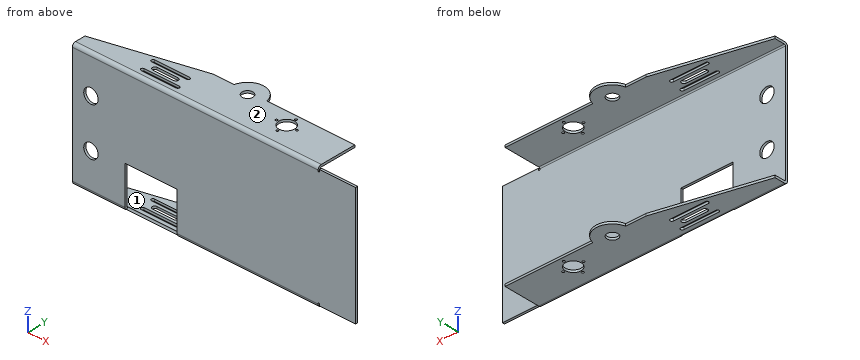
from build123d import *

# Parameters (mm, degrees)
SKETCH3_W                       = 250
SKETCH3_H                       = 105
SKETCH3_R                       = 6.35
BASE_FLANGE1_DEPTH              = 2
EDGE_FLANGE1_STRIP_W            = 10
EDGE_FLANGE1_STRIP_H            = 2
EDGE_FLANGE1_STRIP_CUT_DEPTH    = 217
EDGE_FLANGE1_RELIEF_W           = 11
EDGE_FLANGE1_RELIEF_H           = 1
EDGE_FLANGE1_RELIEF_CUT_DEPTH   = 2
EDGE_FLANGE1_STRIP_2_W          = 10
EDGE_FLANGE1_STRIP_2_H          = 2
EDGE_FLANGE1_STRIP_CUT_2_DEPTH  = 217
EDGE_FLANGE1_RELIEF_2_W         = 11
EDGE_FLANGE1_RELIEF_2_H         = 1
EDGE_FLANGE1_RELIEF_CUT_2_DEPTH = 2
EDGE_FLANGE1_DEPTH              = 217
EDGE_FLANGE1_START              = 2
EDGE_FLANGE1_PROFILE_R          = 4.7625
EDGE_FLANGE1_FLAT_DEPTH         = 2
EDGE_FLANGE1_BEND_DEPTH         = 217
EDGE_FLANGE1_PROFILE_2_R        = 4.7625
EDGE_FLANGE1_FLAT_2_DEPTH       = 2
CUT_EXTRUDE2_START              = -78.75
CUT_EXTRUDE2_DEPTH              = 46.25
CUT_EXTRUDE1_DEPTH              = 144.523278273
CUT_EXTRUDE1_DEPTH_BACK         = 144.523278273
SKETCH14_R                      = 1
SKETCH14_R_2                    = 7


# Read off the part's stored shape, not the designer's step: Cut-Extrude2
# Sheet-metal steps are written as plain solids
with BuildPart() as part:
    # Sketch3 → Base-Flange1 (new body)
    with BuildSketch(Plane(origin=(0, 0, 0), x_dir=(1, 0, 0), z_dir=(0, 1, 0))):
        Rectangle(SKETCH3_W, SKETCH3_H)
        with Locations(Location((-108.65, 21.15, 0), (0, 0, 270))):
            Circle(SKETCH3_R, mode=Mode.SUBTRACT)
        with Locations(Location((-108.65, -21.15, 0), (0, 0, 90))):
            Circle(SKETCH3_R, mode=Mode.SUBTRACT)
    extrude(amount=-BASE_FLANGE1_DEPTH)

    # Edge-Flange1 strip (across the edge) → Edge-Flange1 strip cut (cut)
    with BuildSketch(Plane(origin=(-125, 0, 52.5), x_dir=(0, 0, -1), z_dir=(1, 0, 0))):
        with Locations((-4, -1)):
            Rectangle(EDGE_FLANGE1_STRIP_W, EDGE_FLANGE1_STRIP_H)
    extrude(amount=EDGE_FLANGE1_STRIP_CUT_DEPTH, mode=Mode.SUBTRACT)

    # Edge-Flange1 relief (on the sheet) → Edge-Flange1 relief cut (cut)
    with BuildSketch(Plane(origin=(-125, 0, 51.5), x_dir=(0, 0, -1), z_dir=(0, 1, 0))):
        with Locations((-4.5, -217.5)):
            Rectangle(EDGE_FLANGE1_RELIEF_W, EDGE_FLANGE1_RELIEF_H)
    extrude(amount=-EDGE_FLANGE1_RELIEF_CUT_DEPTH, mode=Mode.SUBTRACT)

    # Edge-Flange1 strip 2 (across the edge) → Edge-Flange1 strip cut 2 (cut)
    with BuildSketch(Plane(origin=(92, 0, -52.5), x_dir=(0, 0, 1), z_dir=(-1, 0, 0))):
        with Locations((-4, -1)):
            Rectangle(EDGE_FLANGE1_STRIP_2_W, EDGE_FLANGE1_STRIP_2_H)
    extrude(amount=EDGE_FLANGE1_STRIP_CUT_2_DEPTH, mode=Mode.SUBTRACT)

    # Edge-Flange1 relief 2 (on the sheet) → Edge-Flange1 relief cut 2 (cut)
    with BuildSketch(Plane(origin=(92, 0, -51.5), x_dir=(0, 0, 1), z_dir=(0, 1, 0))):
        with Locations((-4.5, 0.5)):
            Rectangle(EDGE_FLANGE1_RELIEF_2_W, EDGE_FLANGE1_RELIEF_2_H)
    extrude(amount=-EDGE_FLANGE1_RELIEF_CUT_2_DEPTH, mode=Mode.SUBTRACT)

    # Edge-Flange1 bend section (across the edge) → Edge-Flange1 (add)
    with BuildSketch(Plane(origin=(-125, 0, 52.5), x_dir=(0, 0, -1), z_dir=(1, 0, 0))):
        with BuildLine():
            Line((-2, 1), (0, 1))
            ThreePointArc((0, 1), (0.292893219, 0.292893219), (1, 0))
            Line((1, 0), (1, -2))
            ThreePointArc((1, -2), (-1.121320344, -1.121320344), (-2, 1))
        make_face()
    extrude(amount=EDGE_FLANGE1_DEPTH)

    # Edge-Flange1 profile (on flange) → Edge-Flange1 flat (add)
    with BuildSketch(Plane.XY.offset(52.5).offset(EDGE_FLANGE1_START)):
        with BuildLine():
            Line((-125, 9.993471807), (-125, 1))
            Line((-125, 1), (92, 1))
            Line((92, 1), (92, 33))
            Line((92, 33), (14.454459736, 33))
            ThreePointArc((14.454459736, 33), (0, 44.7625), (-14.454459736, 33))
            Line((-14.454459736, 33), (-32.5, 33))
            Line((-32.5, 33), (-125, 9.993471807))
        make_face()
        with Locations((0, 30)):
            Circle(EDGE_FLANGE1_PROFILE_R, mode=Mode.SUBTRACT)
    extrude(amount=-EDGE_FLANGE1_FLAT_DEPTH)

    # Edge-Flange1 bend section 2 (across the edge) → Edge-Flange1 bend (add)
    with BuildSketch(Plane(origin=(92, 0, -52.5), x_dir=(0, 0, 1), z_dir=(-1, 0, 0))):
        with BuildLine():
            Line((-2, 1), (0, 1))
            ThreePointArc((0, 1), (0.292893219, 0.292893219), (1, 0))
            Line((1, 0), (1, -2))
            ThreePointArc((1, -2), (-1.121320344, -1.121320344), (-2, 1))
        make_face()
    extrude(amount=EDGE_FLANGE1_BEND_DEPTH)

    # Edge-Flange1 profile 2 (on flange) → Edge-Flange1 flat 2 (add)
    with BuildSketch(Plane(origin=(0, 0, -52.5), x_dir=(-1, 0, 0), z_dir=(0, 0, -1)).offset(EDGE_FLANGE1_START)):
        with BuildLine():
            ThreePointArc((14.454459736, 33), (0, 44.7625), (-14.454459736, 33))
            Line((-14.454459736, 33), (-92, 33))
            Line((-92, 33), (-92, 1))
            Line((-92, 1), (125, 1))
            Line((125, 1), (125, 9.993471807))
            Line((125, 9.993471807), (32.5, 33))
            Line((32.5, 33), (14.454459736, 33))
        make_face()
        with Locations((0, 30)):
            Circle(EDGE_FLANGE1_PROFILE_2_R, mode=Mode.SUBTRACT)
    extrude(amount=-EDGE_FLANGE1_FLAT_2_DEPTH)

    # Cut-Extrude2 outline → Cut-Extrude2 (cut)
    with BuildSketch(Plane.YZ.offset(CUT_EXTRUDE2_START)):
        with BuildLine():
            Line((0, -54.328427125), (0.666666667, -52.442809042))
            ThreePointArc((0.666666667, -52.442809042), (0.183503419, -52.077350269), (0, -51.5))
            Line((0, -51.5), (0, -17.5))
            Line((0, -17.5), (-2, -17.5))
            Line((-2, -17.5), (-2, -51.5))
            ThreePointArc((-2, -51.5), (-1.449489743, -53.232050808), (0, -54.328427125))
        make_face()
    extrude(amount=CUT_EXTRUDE2_DEPTH, mode=Mode.SUBTRACT)

    # Sketch14 → Cut-Extrude1 (cut, two sides: drawn at the far end of the back side and taken through both)
    with BuildSketch(Plane.XY.offset(-CUT_EXTRUDE1_DEPTH_BACK)):
        with BuildLine():
            Line((-46.5, 14.125), (-65.166666667, 14.125))
            ThreePointArc((-65.166666667, 14.125), (-67.291666667, 12), (-65.166666667, 9.875))
            Line((-65.166666667, 9.875), (-46.5, 9.875))
            ThreePointArc((-46.5, 9.875), (-44.375, 12), (-46.5, 14.125))
        make_face()
        with BuildLine():
            Line((-57.900010285, 4.380710415), (-51.653085966, 4.380710415))
            ThreePointArc((-51.653085966, 4.380710415), (-50.153085966, 5.880710415), (-51.653085966, 7.380710415))
            Line((-51.653085966, 7.380710415), (-57.900010285, 7.380710415))
            ThreePointArc((-57.900010285, 7.380710415), (-59.400010285, 5.880710415), (-57.900010285, 4.380710415))
        make_face()
        with BuildLine():
            Line((-51.653085966, 4.380710415), (-39.233343618, 4.380710415))
            ThreePointArc((-39.233343618, 4.380710415), (-37.733343618, 5.880710415), (-39.233343618, 7.380710415))
            Line((-39.233343618, 7.380710415), (-51.653085966, 7.380710415))
            ThreePointArc((-51.653085966, 7.380710415), (-50.153085966, 5.880710415), (-51.653085966, 4.380710415))
        make_face()
        with BuildLine():
            Line((-70.319752633, 4.380710415), (-57.900010285, 4.380710415))
            ThreePointArc((-57.900010285, 4.380710415), (-59.400010285, 5.880710415), (-57.900010285, 7.380710415))
            Line((-57.900010285, 7.380710415), (-70.319752633, 7.380710415))
            ThreePointArc((-70.319752633, 7.380710415), (-71.819752633, 5.880710415), (-70.319752633, 4.380710415))
        make_face()
        with BuildLine():
            Line((-72.433323049, 16.619289585), (-60.0135807, 16.619289585))
            ThreePointArc((-60.0135807, 16.619289585), (-61.5135807, 18.119289585), (-60.0135807, 19.619289585))
            Line((-60.0135807, 19.619289585), (-72.433323049, 19.619289585))
            ThreePointArc((-72.433323049, 19.619289585), (-73.933323049, 18.119289585), (-72.433323049, 16.619289585))
        make_face()
        with BuildLine():
            Line((-60.0135807, 16.619289585), (-53.766656382, 16.619289585))
            ThreePointArc((-53.766656382, 16.619289585), (-52.266656382, 18.119289585), (-53.766656382, 19.619289585))
            Line((-53.766656382, 19.619289585), (-60.0135807, 19.619289585))
            ThreePointArc((-60.0135807, 19.619289585), (-61.5135807, 18.119289585), (-60.0135807, 16.619289585))
        make_face()
        with BuildLine():
            ThreePointArc((-53.766656382, 19.619289585), (-52.266656382, 18.119289585), (-53.766656382, 16.619289585))
            Line((-53.766656382, 16.619289585), (-41.346914034, 16.619289585))
            ThreePointArc((-41.346914034, 16.619289585), (-39.846914034, 18.119289585), (-41.346914034, 19.619289585))
            Line((-41.346914034, 19.619289585), (-53.766656382, 19.619289585))
        make_face()
        with Locations((43.5, 11.4)):
            Circle(SKETCH14_R)
        with Locations((52.5, 20.4)):
            Circle(SKETCH14_R)
        with Locations((43.5, 20.4)):
            Circle(SKETCH14_R_2)
        with Locations((34.5, 20.4)):
            Circle(SKETCH14_R)
        with Locations((43.5, 29.4)):
            Circle(SKETCH14_R)
    extrude(amount=CUT_EXTRUDE1_DEPTH + CUT_EXTRUDE1_DEPTH_BACK, mode=Mode.SUBTRACT)


solid = part.part
The listing builds one solid part. Answer for the finished solid, in the listing's coordinates (mm). Face numbers are marked on the shaded views. A direction names the side the tool comes from. Give positions to 0.01 mm unless a question says otherwise; leave off trailing zeros. Write each loop counter-clockwise with the first axis right and the second up, starting at its lowest first coordinate (ties: lowest second). Pieces come first, ordered by that corner, then holes.
1) Section A-A (z = -21.15) is taken. Write down the section's boundary in (x, y), and give its area (3 significant figures).
2) Section C-C (x = 0) is taken. Write down the section's boundary in (y, z).
3) Section D-D (z = -38.5) is taken. Write down the section's boundary in (x, y).
4) Find the intervals of material crossed by L1, parallel to X at y = -0.5, z = 21.15; L2, parallel to Z at x = -2.5, y = 36.5; L3, parallel to Y at x = -15.5, z = 11.5, in increasing order.
5) A tool of negligible diameter and unlimited length cuts with its end or side. For the marked faces 1 and 2, from which of +Z, -Z, +X, -X, +Y, -Y can it reach the whole face along a straight path? Write none if from no direction.
6) Given P1, Ø4.5, axis at y = 22.5, z = -52.5, coming from the +X side; P2, Ø1.6, axis at x = -58, z = -54, coming from the +Y side; P3, Ø1, axis at x = -53.5, z = -53, coming from the -Y side, each flat-ended and moving along its own axis, determine where each tip first touches the part or whether it passes through.
7) Section B-B (z = 21.15) is taken. Write down the section's boundary in (x, y), and give its area (3 significant figures).
Response:
1. outline: (-125, -2) - (-115, -2) - (-115, 0) - (-125, 0) - close; (-102.3, -2) - (-78.75, -2) - (-78.75, 0) - (-102.3, 0) - close; (-32.5, -2) - (125, -2) - (125, 0) - (-32.5, 0) - close
1. area: 382 mm2
2. outline: (-2, -51.5) arc R3 ccw to (1, -54.5) - (25.24, -54.5) - (25.24, -52.5) - (1, -52.5) arc R1 cw to (0, -51.5) - (0, 51.5) arc R1 cw to (1, 52.5) - (25.24, 52.5) - (25.24, 54.5) - (1, 54.5) arc R3 ccw to (-2, 51.5) - close; (34.76, -54.5) - (44.76, -54.5) - (44.76, -52.5) - (34.76, -52.5) - close; (34.76, 52.5) - (44.76, 52.5) - (44.76, 54.5) - (34.76, 54.5) - close
3. outline: (-125, -2) - (-78.75, -2) - (-78.75, 0) - (-125, 0) - close; (-32.5, -2) - (125, -2) - (125, 0) - (-32.5, 0) - close
4. L1: x = -125 to -115, -102.3 to 125
4. L2: z = -54.5 to -52.5, 52.5 to 54.5
4. L3: y = -2 to 0
5. face 1: +X, -X, +Y
5. face 2: +Z, +X, -X, +Y, -Y
6. P1: stops at x = 92
6. P2: stops at y = 26.86
6. P3: stops at y = 0.29
7. outline: (-125, -2) - (-115, -2) - (-115, 0) - (-125, 0) - close; (-102.3, -2) - (125, -2) - (125, 0) - (-102.3, 0) - close
7. area: 475 mm2
